Verification items for the finished model (mm, model axes). Face numbers are marked on the shaded views. A direction names the side the tool comes from. Give positions to 0.01 mm unless a question says otherwise; leave off trailing zeros. Write each loop counter-clockwise with the first axis right and the second up, starting at its lowest first coordinate (ties: lowest second). Pieces come first, ordered by that corner, then holes. Notation, with made-up numbers: M -15,53.5 L 10,53.5 A22 ccw 10,76.5 Z; hole C -25,30 d2. An arc over 180 degrees is marked long. Write item = value, one per line.
Autodesk Inventor part; units mm, degrees
ref_plane "YZ Plane" through (0, 0, 0) normal (1, 0, 0) x (0, 1, 0)
ref_plane "XZ Plane" through (0, 0, 0) normal (0, 1, 0) x (-1, 0, 0)
ref_plane "XY Plane" through (0, 0, 0) normal (0, 0, 1) x (1, 0, 0)
sketch "Sketch1" plane through (0, 0, 0) normal (0, 1, 0) x (-1, 0, 0)
  circle A0 centre (0, 0) radius 8.2
  dimension "d0" = 16.4
extrude "Extrusion1" add sketch "Sketch1" along normal blind 33
sketch "Sketch3" plane through (0, 33, 0) normal (0, 1, 0) x (1, 0, 0)
  circle A0 centre (0, 0) radius 11
  dimension "d4" = 22
extrude "Extrusion2" add sketch "Sketch3" along normal blind 3
sketch "Sketch4" plane through (0, 36, 0) normal (0, 1, 0) x (1, 0, 0)
  circle A0 centre (0, 0) radius 1.6
  dimension "d7" = 3.2
extrude "Extrusion3" cut sketch "Sketch4" against normal blind 100
sketch "Sketch5" plane through (0, 36, 0) normal (0, 1, 0) x (1, 0, 0)
  circle A0 centre (0, 0) radius 1.6
  circle A1 centre (0, 0) radius 4
  dimension "d10" = 8
extrude "Extrusion4" cut sketch "Sketch5" against normal blind 3
fillet "Fillet1" radius 2 1 edges at (-11, 36, 0)
properties part number "Foam_wing_mount_bolt"
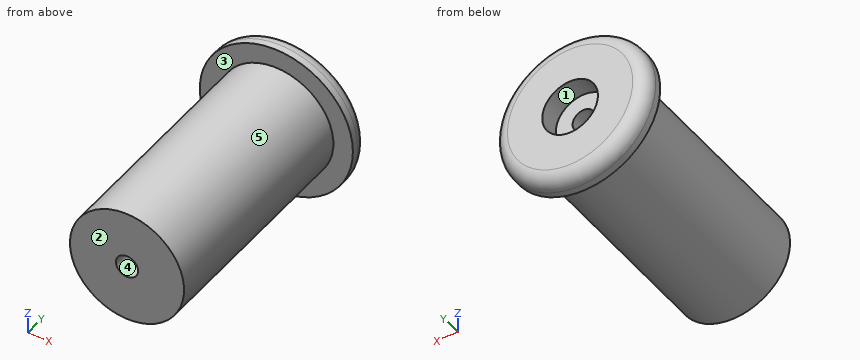
1) Depth check by flat-ended pin: P1, Ø1, axis at y = 16, z = 1.5, coming from the -X side; P2, Ø12, axis at x = -3, y = 14, coming from the -Z side; P3, Ø5, axis at x = -5, y = 11, coming from the +Z side. Enter the tip coordinate at first touch or a pass-through.
From the geometry:
P1 = -8.14
P2 = -8.2
P3 = 7.81
2) Cross-section at A-A on x = 0. Record the boundary of the cut face in (y, z).
From the geometry:
outline = M 0,-8.2 L 33,-8.2 L 33,-11 L 34,-11 A2 ccw 36,-9 L 36,-4 L 33,-4 L 33,-1.6 L 0,-1.6 Z; M 0,1.6 L 33,1.6 L 33,4 L 36,4 L 36,9 A2 ccw 34,11 L 33,11 L 33,8.2 L 0,8.2 Z
3) Cross-section at B-B on z = 0. Record the boundary of the cut face in (x, y).
From the geometry:
outline = M -11,33 L -8.2,33 L -8.2,0 L -1.6,0 L -1.6,33 L -4,33 L -4,36 L -9,36 A2 ccw -11,34 Z; M 1.6,0 L 8.2,0 L 8.2,33 L 11,33 L 11,34 A2 ccw 9,36 L 4,36 L 4,33 L 1.6,33 Z
4) Tool access check on the marked faces 1 and 2. Record the directions out of +Z, -Z, +X, -X, +Y, -Y that give a thin tool (end or side, any length) a straight path to the whole face; none if there is none.
From the geometry:
face_1 = +Y
face_2 = +Z, -Z, +X, -X, -Y
5) Material ranges on probe 1 along Z at (x, y) = (0, 16); probe 2 along X at (y, z) = (34.2, 0); probe 3 along Z at (x, y) = (0, 33.7), recorded low to high. Write a range as from..to.
From the geometry:
probe_1 = -8.2..-1.6, 1.6..8.2
probe_2 = -10.99..-4, 4..10.99
probe_3 = -11..-4, 4..11
6) Cross-section at C-C on y = 28. Record the boundary of the cut face in (x, z).
From the geometry:
outline = C 0,0 d16.4; hole C 0,0 d3.2
7) Draft check along X on the marked faces 3, 4 and 5. Enter one of: +X half, -X half, draft (parallel to the pull), parting line (faces both ways), or undercut.
From the geometry:
face_3 = draft
face_4 = undercut
face_5 = parting line
